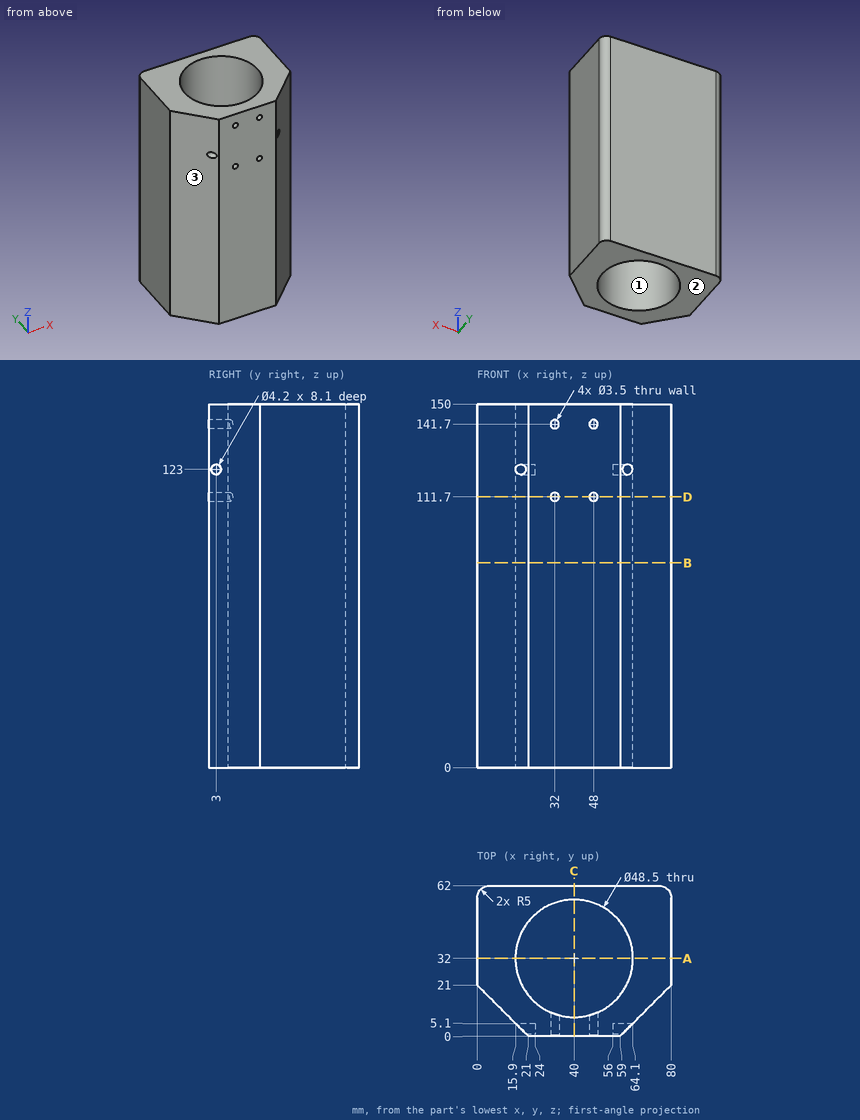
Geometry check sheet. Reference: drawing and pictorial views, mm from the part's lowest x, y, z. Give positions to 0.01 mm unless a question says otherwise; leave off trailing zeros. Write each loop counter-clockwise with the first axis right and the second up, starting at its lowest first coordinate (ties: lowest second). Pieces come first, ordered by that corner, then holes. Notation, with made-up numbers: (72, 43) -> (95, 43) arc R31 cw to (95, 69) -> close; hole circle Ø8 at (52, -5.75). An arc over 180 degrees is marked (long way). One line per question, with ' | ' between items.
Item 1: Sectioned sample at A-A, the plane y = 32. Record the boundary of the cut face in (x, z).
Determined:
outline: (0, 0) -> (15.75, 0) -> (15.75, 150) -> (0, 150) -> close; (64.25, 0) -> (80, 0) -> (80, 150) -> (64.25, 150) -> close
Item 2: Sectioned sample at D-D, the plane z = 111.7. Record the boundary of the cut face in (x, y), plus the area to 3 significant figures.
Determined:
outline: (0, 21) -> (21, 0) -> (30.25, 0) -> (30.25, 9.8) arc R24.25 cw (long way) to (49.75, 9.8) -> (49.75, 0) -> (59, 0) -> (80, 21) -> (80, 57) arc R5 ccw to (75, 62) -> (5, 62) arc R5 ccw to (0, 57) -> close; (33.75, 0) -> (46.25, 0) -> (46.25, 8.57) arc R24.25 cw to (33.75, 8.57) -> close | area: 2,600 mm^2
Item 3: Sectioned sample at C-C, the plane x = 40. Record the boundary of the cut face in (y, z), plus the area to 4 significant figures.
Determined:
outline: (0, 0) -> (7.75, 0) -> (7.75, 150) -> (0, 150) -> close; (56.25, 0) -> (62, 0) -> (62, 150) -> (56.25, 150) -> close | area: 2,025 mm^2
Item 4: Draft check along X on the marked faces 1, 2 and 3. Enter one of: released by +X, released by -X, zero draft, split by the parting line, or undercut.
Determined:
face 1: undercut | face 2: zero draft | face 3: released by -X
Item 5: Depth check by flat-ended pin: pin 1 (5 mm diameter, centred on y = 3, z = 123, fed in from -X); pin 2 (6.5 mm diameter, centred on y = 3, z = 123, fed in from -X); pin 3 (3 mm diameter, centred on x = 32, z = 111.7, fed in from -Y). Enter the tip coordinate at first touch or a pass-through.
Determined:
pin 1: x = 15.5 | pin 2: x = 14.75 | pin 3: y = 54.31
Item 6: Scan lines: line 1 along Z through (x, y) = (32, 8); line 2 along Y through (x, z) = (40, 88); line 3 along Y through (x, z) = (58, 122). Record each from-to range of solid material in increasing order.
Determined:
line 1: 0 to 109.95, 113.45 to 139.95, 143.45 to 150 | line 2: 0 to 7.75, 56.25 to 62 | line 3: 0 to 1.15, 4.85 to 15.75, 48.25 to 62
Item 7: Sectioned sample at B-B, the plane z = 84.5. Record the boundary of the cut face in (x, y).
Determined:
outline: (0, 21) -> (21, 0) -> (59, 0) -> (80, 21) -> (80, 57) arc R5 ccw to (75, 62) -> (5, 62) arc R5 ccw to (0, 57) -> close; hole circle Ø48.5 at (40, 32)
